from build123d import *

# Parameters (mm, degrees)
SKETCH2_W             = 152.4
SKETCH2_H             = 152.4
BOSS_EXTRUDE1_DEPTH   = 1.5875
F_3_0MM_DOWEL_HOLE1_D = 3
F_3_0MM_DOWEL_HOLE2_D = 3
LPATTERN1_COUNT       = 4
LPATTERN1_PITCH       = 42.333333333
LPATTERN2_COUNT       = 4
LPATTERN2_PITCH       = 41.275
SKETCH12_W            = 38.1
SKETCH12_H            = 63.5
CUT_EXTRUDE1_DEPTH    = 2.54
FILLET2_R             = 2.54
SKETCH13_W            = 9.75
SKETCH13_H            = 41.28
CUT_EXTRUDE2_DEPTH    = 216.531993347
SKETCH14_R            = 1.5
CUT_EXTRUDE3_DEPTH    = 10


with BuildPart() as part:
    # Sketch2 → Boss-Extrude1 (new body)
    with BuildSketch(Plane(origin=(0, 0, 0), x_dir=(1, 0, 0), z_dir=(0, 1, 0))):
        with Locations((76.2, 76.2)):
            Rectangle(SKETCH2_W, SKETCH2_H)
    extrude(amount=BOSS_EXTRUDE1_DEPTH)

    # Ø3.0mm Dowel Hole1 (through all)
    with Locations(Plane(origin=(0, 1.5875, 0), x_dir=(1, 0, 0), z_dir=(0, 1, 0))):
        with Locations((14.2875, 147.6375), (14.2875, 4.7625)):
            f_3_0mm_dowel_hole1 = Hole(F_3_0MM_DOWEL_HOLE1_D / 2)

    # Ø3.0mm Dowel Hole2 (through all)
    with Locations(Plane(origin=(0, 1.5875, 0), x_dir=(1, 0, 0), z_dir=(0, 1, 0))):
        with Locations((4.7625, 139.7), (147.6375, 139.7)):
            f_3_0mm_dowel_hole2 = Hole(F_3_0MM_DOWEL_HOLE2_D / 2)

    # LPattern1: Ø3.0mm Dowel Hole2 ×4, 1 skipped
    with Locations(*[(0, 0, i * LPATTERN1_PITCH) for i in range(1, LPATTERN1_COUNT) if i not in (1,)]):
        add(f_3_0mm_dowel_hole2, mode=Mode.SUBTRACT)

    # LPattern2: Ø3.0mm Dowel Hole1 ×4
    with Locations(*[(i * LPATTERN2_PITCH, 0, 0) for i in range(1, LPATTERN2_COUNT)]):
        add(f_3_0mm_dowel_hole1, mode=Mode.SUBTRACT)

    # Sketch12 → Cut-Extrude1 (cut)
    with BuildSketch(Plane(origin=(0, 1.5875, 0), x_dir=(1, 0, 0), z_dir=(0, 1, 0))):
        with Locations((76.2, 88.9)):
            Rectangle(SKETCH12_W, SKETCH12_H)
    extrude(amount=-CUT_EXTRUDE1_DEPTH, mode=Mode.SUBTRACT)

    # Fillet2
    fillet2_edges = [part.edges().sort_by_distance(p)[0] for p in [
        (95.25, 0.79375, -120.65),
        (95.25, 0.79375, -57.15),
        (57.15, 0.79375, -57.15),
        (57.15, 0.79375, -120.65),
    ]]
    fillet(fillet2_edges, radius=FILLET2_R)

    # Sketch13 → Cut-Extrude2 (cut, through all)
    with BuildSketch(Plane(origin=(0, 1.5875, 0), x_dir=(1, 0, 0), z_dir=(0, 1, 0))):
        with Locations((147.525, 88.5)):
            Rectangle(SKETCH13_W, SKETCH13_H)
        with Locations((4.875, 88.5)):
            Rectangle(SKETCH13_W, SKETCH13_H)
    extrude(amount=-CUT_EXTRUDE2_DEPTH, mode=Mode.SUBTRACT)

    # Sketch14 → Cut-Extrude3 (cut)
    with BuildSketch(Plane.XZ):
        with Locations(Location((120.450623047, -40.719396702, 0), (0, 0, 270))):
            Circle(SKETCH14_R)
        with Locations(Location((106.400623047, -40.719396702, 0), (0, 0, 270))):
            Circle(SKETCH14_R)
        with Locations(Location((106.400623047, -70.719396702, 0), (0, 0, 270))):
            Circle(SKETCH14_R)
        with Locations(Location((120.450623047, -70.719396702, 0), (0, 0, 270))):
            Circle(SKETCH14_R)
    extrude(amount=-CUT_EXTRUDE3_DEPTH, mode=Mode.SUBTRACT)


solid = part.part
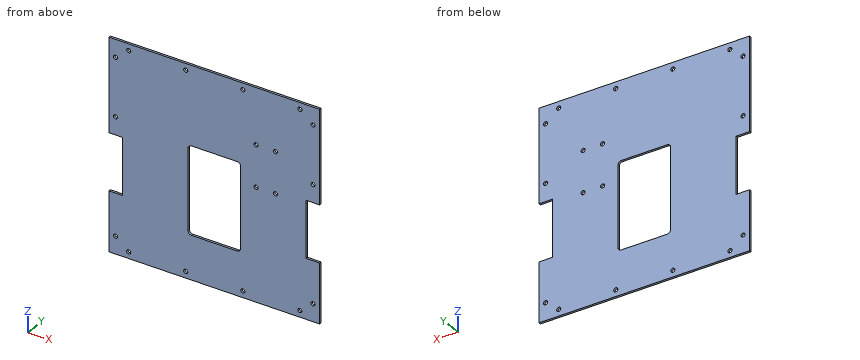
Model file for the job. Use its own axes, mm. Give positions to 0.01 mm unless a question says otherwise; leave off trailing zeros. Order: outer loops, then holes, each group sorted by start corner. A loop starts at its lowest first (then second) coordinate and runs counter-clockwise, first axis right, second up. Notation, with made-up numbers: M 11,-36.5 L 54,-36.5 A20 cw 54,-8.5 Z; hole C 89,-25 d6. An arc over 180 degrees is marked long. Put each result on its own line as item: value. Start each with the question number.
(1) Band-saw the part on A-A on z = -92.5. Give the cut face in (x, y).
(2) Drill centre lines: L1, parallel to X at y = 0.8, z = -139.7; L2, parallel to X at y = 1.45, z = -70.5; L3, parallel to X at y = 0.5, z = -88. Where is each one in solid material? Low to high. Write a range as [from, to].
(3) Pin check, flat tips, straight feed: pin 1 Ø2.5 at (x, z) = (4.76, -55.03) entering from +Y; pin 2 Ø0.5 at (y, z) = (0.5, -82.5) entering from +X. Stop position of each tip, or through.
(4) Band-saw the part on B-B on y = 0.4. Count the separate pieces of the cut face and the enclosed holes in it, then the cut area to 3 significant figures.
Results below:
1. outline: M 9.75,0 L 57.15,0 L 57.15,1.59 L 9.75,1.59 Z; M 95.25,0 L 142.65,0 L 142.65,1.59 L 95.25,1.59 Z
2. L1: x = [0, 3.26], [6.26, 146.14], [149.14, 152.4]
2. L2: x = [9.75, 57.15], [95.25, 104.92], [107.88, 118.97], [121.93, 142.65]
2. L3: x = [9.75, 57.15], [95.25, 142.65]
3. pin 1: passes through
3. pin 2: stops at x = 142.65
4. separate pieces: 1
4. enclosed holes: 19
4. area: 19,900 mm2
